Geometry check sheet. Reference: the model listing, model coordinates, mm. A direction names the side the tool comes from. Round coordinates to 2 decimals unless told otherwise and drop trailing zeros. Loops run counter-clockwise (first coordinate to the right, second up) from the corner with the lowest first, then second, coordinate; pieces in that order, holes last. Notation, with made-up numbers: (53, -26.75) -> (67, -26.75) arc R22 ccw to (67, -7.75) -> close; hole circle Ø11 at (14.25, 64). An arc over 180 degrees is marked (long way). Use a Markdown table: item, result. Add a question column.
Q1. Set-up check for faces 1 (the face through (-23, -3.5, 1)), 2 (the face through (-23, 3.5, 1)), 3 (the face through (-4.725, -0.031, 1.479)): record each of +Z, -Z, +X, -X, +Y, -Y from which the full face is reachable in a straight line by a thin tool's end or side.
Q2. Gauge pin test, flat ends, axial feed: P1, Ø0.8, axis at x = -23.5, z = 2, coming from the -Y side; P2, Ø6, axis at x = 2.5, y = 3.5, coming from the -Z side; P3, Ø1.5, axis at y = 5.5, z = 1, coming from the +X side; P4, Ø0.8, axis at x = -23, z = 1.5, coming from the +Y side. Record the tip position at first contact, or that the pin passes through.
Q3. Material ranges on L1, parallel to X at y = 3.25, z = 2.2; L2, parallel to X at y = -4.75, z = 2; L3, parallel to X at y = 5.25, z = 0.3, recorded low to high.
Q4. Sectioned sample at B-B, the plane y = -6.5. Enter the section's corners in (x, z).
Q5. Sectioned sample at A-A, the plane x = -3. Enter the section's corners in (y, z).
Q6. Release check for a two-part mould opening along X. For faces 4 (the face through (7.8, -6, 1)), 5 (the face through (-3.204, -6.136, 1.479)), 6 (the face through (6, -8, 1)) record: released by +X, released by -X, zero draft, split by the parting line, or undercut.
```python
from build123d import *

# Parameters (mm, degrees)
BOSS_EXTRU_1_DEPTH = 3


with BuildPart() as part:
    # Esquisse1 → Boss.-Extru.1 (new body)
    with BuildSketch(Plane.XY):
        with BuildLine():
            Line((-24.7, -3.5), (-22.2, -3.5))
            Line((-22.2, -3.5), (-22.2, -8))
            Line((-22.2, -8), (-3.993420642, -8))
            Line((-3.993420642, -8), (-2.392209052, -4.218369106))
            ThreePointArc((-2.392209052, -4.218369106), (-2.646725452, -2.729399825), (-4.10580345, -2.338376153))
            ThreePointArc((-4.10580345, -2.338376153), (-4.724999134, 0.00286091), (-4.102968743, 2.343346431))
            ThreePointArc((-4.102968743, 2.343346431), (-2.687005769, 2.687005769), (-2.343346431, 4.102968743))
            ThreePointArc((-2.343346431, 4.102968743), (0, 4.725), (2.343346431, 4.102968743))
            ThreePointArc((2.343346431, 4.102968743), (2.687005769, 2.687005769), (4.102968743, 2.343346431))
            ThreePointArc((4.102968743, 2.343346431), (4.724999134, 0.00286091), (4.10580345, -2.338376153))
            ThreePointArc((4.10580345, -2.338376153), (2.646725452, -2.729399825), (2.392209052, -4.218369106))
            Line((2.392209052, -4.218369106), (3.993420642, -8))
            Line((3.993420642, -8), (7.8, -8))
            Line((7.8, -8), (7.8, -3.5))
            Line((7.8, -3.5), (10.3, -3.5))
            Line((10.3, -3.5), (10.3, 3.5))
            Line((10.3, 3.5), (7.8, 3.5))
            Line((7.8, 3.5), (7.8, 8))
            Line((7.8, 8), (-22.2, 8))
            Line((-22.2, 8), (-22.2, 3.5))
            Line((-22.2, 3.5), (-24.7, 3.5))
            Line((-24.7, 3.5), (-24.7, -3.5))
        make_face()
    extrude(amount=BOSS_EXTRU_1_DEPTH)


solid = part.part
```
Values:
| question | item | result |
|---|---|---|
| 1 | face 1 | +Z, -Z, -X, -Y |
| 1 | face 2 | +Z, -Z, -X, +Y |
| 1 | face 3 | +Z, -Z |
| 2 | P1 | y = -3.5 |
| 2 | P2 | z = 0 |
| 2 | P3 | x = 7.8 |
| 2 | P4 | y = 3.5 |
| 3 | L1 | -24.7 to -2.34, 2.34 to 10.3 |
| 3 | L2 | -22.2 to -2.62, 2.62 to 7.8 |
| 3 | L3 | -22.2 to 7.8 |
| 4 | outline | (-22.2, 0) -> (-3.36, 0) -> (-3.36, 3) -> (-22.2, 3) -> close; (3.36, 0) -> (7.8, 0) -> (7.8, 3) -> (3.36, 3) -> close |
| 5 | outline | (-5.65, 0) -> (-2.45, 0) -> (-2.45, 3) -> (-5.65, 3) -> close; (2.45, 0) -> (8, 0) -> (8, 3) -> (2.45, 3) -> close |
| 6 | face 4 | released by +X |
| 6 | face 5 | undercut |
| 6 | face 6 | zero draft |
